The figure shows three views and two pictorial views of one solid part (mm, origin at its lowest corner). Answer the questions. Coordinates: 2 decimals unless noted, no trailing zeros. Order: outer loops, then holes, each group sorted by start corner. A loop starts at its lowest first (then second) coordinate and runs counter-clockwise, first axis right, second up. Notation, with made-up numbers: (62.5, 70.5) -> (86.5, 70.5) arc R25 ccw to (86.5, 106.5) -> close; hole circle Ø11 at (82.25, 0.5). An arc over 180 degrees is marked (long way). Use one line per item in the form item = value.
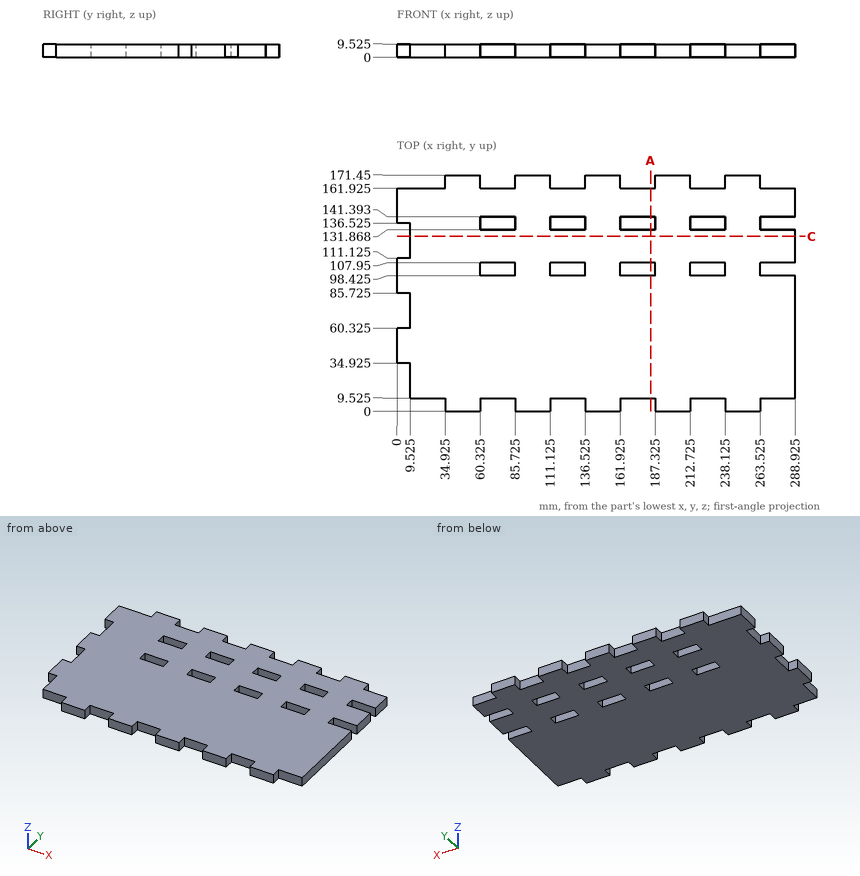
(1) Section C-C on y = 127 is taken. Write down the section's boundary in (x, z) (3 decimals).
Data:
outline = (9.525, 0) -> (288.925, 0) -> (288.925, 9.525) -> (9.525, 9.525) -> close
(2) Straight lines are drawn through the part: line 1 along X through (y, z) = (8, 6) (3 decimals); line 2 along X through (y, z) = (107, 5) (3 decimals); line 3 along X through (y, z) = (129.5, 6.75) (3 decimals). For each, find the intervals that lie inside material, in ascending order.
Data:
line_1 = 34.925 to 60.325, 85.725 to 111.125, 136.525 to 161.925, 187.325 to 212.725, 238.125 to 263.525
line_2 = 0 to 60.325, 85.725 to 111.125, 136.525 to 161.925, 187.325 to 212.725, 238.125 to 263.525
line_3 = 9.525 to 288.925
(3) Each of these flat-tipped pins is pushed along its axis until it touches: P1, Ø5, axis at x = 79, z = 5.5, coming from the +Y side (3 decimals); P2, Ø1.5, axis at y = 102.5, z = 4, coming from the +X side (3 decimals); P3, Ø3, axis at x = 279, z = 7, coming from the -Y side (3 decimals). Where does it stop, or does it pass through?
Data:
P1 = 161.925
P2 = 263.525
P3 = 9.525
(4) Section A-A on x = 184 is taken. Count the separate pieces of the cut face and the enclosed holes in it, plus the area to 3 significant figures.
Data:
separate_pieces = 3
enclosed_holes = 0
area = 1,270 mm²
